Input: part model. Units: mm. Frame: model coordinates. A direction names the side the tool comes from. Round coordinates to 2 decimals unless told otherwise and drop trailing zeros. Loops run counter-clockwise (first coordinate to the right, second up) from the corner with the lowest first, then second, coordinate; pieces in that order, holes last. Notation, with made-up numbers: (1.5, 8.5) - (21.5, 8.5) arc R16 ccw to (21.5, 34.5) - close; hole circle Ø6 at (22.5, -4.75). An arc over 180 degrees is marked (long way). Use CSV: the item, a comma, the result in double quotes. Start each with the question number.
1. Pull-direction query (X, two-part tool) for faces 3 (the flat face through (2, 2, 9.5)), 4 (the cylindrical face through (-2.17, -9.76, 1.48)), 5 (the cylindrical face through (4.03, -3.18, 1.48)); classes: +X half, -X half, draft (parallel to the pull), parting line (faces both ways), or undercut.
2. Material intervals for probe 1 along Y at (x, z) = (0, 1.3); probe 2 along Y at (x, z) = (6, 1.75); probe 3 along Z at (x, y) = (-4.75, 0), sorted ascending. Write a range as from..to.
3. Access query for faces 1 (the cylindrical face through (-0.867, -3.905, 6.204)), 2 (the flat face through (2, -2, 0)). Directions: +Z, -Z, +X, -X, +Y, -Y. A direction counts if a zero-diameter tool reaches every point of the face in a straight line with its end or side. Return the directions, or none.
4. Pin query (flat end, axial travel): P1, Ø2.5, axis at x = -5.63, y = -3.25, coming from the +Z side; P2, Ø2, axis at x = 5, z = 2, coming from the +Y side; P3, Ø4, axis at x = 7, z = 4.5, coming from the +Y side. Return the tip coordinate at first contact, or that it passes through.
5. Cut plane A-A (y = 0). Return loops of the section in (x, z), and give its area (3 significant figures).
6. Cut plane D-D (z = 7). Return loops of the section in (x, y), and give its area (3 significant figures).
7. Cut plane C-C (x = -2). Return loops of the section in (y, z).
8. Cut plane B-B (x = 0). Return loops of the section in (y, z), and give its area (3 significant figures).
```python
from build123d import *

# Parameters (mm, degrees)
F2_R     = 10
F2_R_2   = 1.6
F2_R_3   = 4
F2_R_4   = 2.5
F3_DEPTH = 3
F4_DEPTH = 9.5


with BuildPart() as f3:
    # F2 (on Top) → F3 (new body)
    with BuildSketch(Plane.XY):
        Circle(F2_R)
        with Locations((-5.6291651246, -3.25)):
            Circle(F2_R_2, mode=Mode.SUBTRACT)
        with Locations((5.6291651246, -3.25)):
            Circle(F2_R_2, mode=Mode.SUBTRACT)
        Circle(F2_R_3, mode=Mode.SUBTRACT)
        with Locations((0, 6.5)):
            Circle(F2_R_2, mode=Mode.SUBTRACT)
        Circle(F2_R_3)
        Circle(F2_R_4, mode=Mode.SUBTRACT)
    extrude(amount=F3_DEPTH)

    # F2 (on Top) → F4 (join)
    with BuildSketch(Plane.XY):
        Circle(F2_R_3)
        Circle(F2_R_4, mode=Mode.SUBTRACT)
    extrude(amount=F4_DEPTH)


solid = f3.part
```
Established:
1,face 3,"draft"
1,face 4,"parting line"
1,face 5,"undercut"
2,probe 1,"y = -10..-2.5, 2.5..4.9, 8.1..10"
2,probe 2,"y = -8..-4.81, -1.69..8"
2,probe 3,"z = 0..3"
3,face 1,"+Z"
3,face 2,"-Z, +X, -X, +Y, -Y"
4,P1,"passes through"
4,P2,"stops at y = 9.17"
4,P3,"stops at y = 8.23"
5,outline,"(-10, 0) - (-2.5, 0) - (-2.5, 9.5) - (-4, 9.5) - (-4, 3) - (-10, 3) - close; (2.5, 0) - (10, 0) - (10, 3) - (4, 3) - (4, 9.5) - (2.5, 9.5) - close"
5,area,"64.5 mm2"
6,outline,"circle Ø8 at (0, 0); hole circle Ø5 at (0, 0)"
6,area,"30.6 mm2"
7,outline,"(-9.8, 0) - (-1.5, 0) - (-1.5, 9.5) - (-3.46, 9.5) - (-3.46, 3) - (-9.8, 3) - close; (1.5, 0) - (9.8, 0) - (9.8, 3) - (3.46, 3) - (3.46, 9.5) - (1.5, 9.5) - close"
8,outline,"(-10, 0) - (-2.5, 0) - (-2.5, 9.5) - (-4, 9.5) - (-4, 3) - (-10, 3) - close; (2.5, 0) - (4.9, 0) - (4.9, 3) - (4, 3) - (4, 9.5) - (2.5, 9.5) - close; (8.1, 0) - (10, 0) - (10, 3) - (8.1, 3) - close"
8,area,"54.9 mm2"
